For this review, take the finished solid that the model builds, in its own axes (mm). A direction names the side the tool comes from. Coordinates: 2 decimals unless noted, no trailing zeros. Loops run counter-clockwise (first coordinate to the right, second up) from the corner with the lowest first, then second, coordinate; pieces in that order, holes last. Notation, with made-up numbers: (-30.5, -0.5) -> (-18.5, -0.5) arc R16 cw to (-18.5, 16.5) -> close; hole circle Ø7 at (-13, -16.5). An arc over 180 degrees is marked (long way). Answer in a Markdown table with one row per item.
from build123d import *

# Parameters (mm, degrees)
SKETCH1_W           = 99.7966
SKETCH1_H           = 30.1244
BOSS_EXTRUDE1_DEPTH = 2.54
SKETCH2_W           = 33.65475448
SKETCH2_H           = 6.70026545
BOSS_EXTRUDE2_DEPTH = 10.16
SKETCH3_R           = 5.045566178
SKETCH3_W           = 25.4
SKETCH3_H           = 25.4
BOSS_EXTRUDE3_DEPTH = 3.556
FILLET1_R           = 2.54
SKETCH4_R           = 3.429
BOSS_EXTRUDE4_DEPTH = 2.54
FILLET2_R           = 2.54
CHAMFER1_SIZE       = 2.38
SKETCH5_W           = 0.314102564
SKETCH5_H           = 3.5
CUT_EXTRUDE1_DEPTH  = 0.762


with BuildPart() as part:
    # Sketch1 → Boss-Extrude1 (new body)
    with BuildSketch(Plane(origin=(0, 0, 0), x_dir=(1, 0, 0), z_dir=(0, 1, 0))):
        with Locations((49.8983, 15.0622)):
            Rectangle(SKETCH1_W, SKETCH1_H)
    extrude(amount=BOSS_EXTRUDE1_DEPTH)

    # Sketch2 → Boss-Extrude2 (add)
    with BuildSketch(Plane(origin=(0, 2.54, 0), x_dir=(1, 0, 0), z_dir=(0, 1, 0))):
        with Locations((30.013421746, 3.350132725)):
            Rectangle(SKETCH2_W, SKETCH2_H)
    extrude(amount=BOSS_EXTRUDE2_DEPTH)

    # Sketch3 → Boss-Extrude3 (add)
    with BuildSketch(Plane(origin=(0, 2.54, 0), x_dir=(1, 0, 0), z_dir=(0, 1, 0))):
        with Locations(Location((37.834363192, 18.707427202, 0), (0, 0, 90))):
            Circle(SKETCH3_R)
        with Locations((79.4766, 15.0622)):
            Rectangle(SKETCH3_W, SKETCH3_H)
    extrude(amount=BOSS_EXTRUDE3_DEPTH)

    # Fillet1
    fillet1_edges = [part.edges().sort_by_distance(p)[0] for p in [
        (92.1766, 4.318, -27.7622),
        (66.7766, 4.318, -27.7622),
        (66.7766, 4.318, -2.3622),
        (92.1766, 4.318, -2.3622),
    ]]
    fillet(fillet1_edges, radius=FILLET1_R)

    # Sketch4 → Boss-Extrude4 (add)
    with BuildSketch(Plane.ZY):
        with Locations((-15.0622, 0)):
            Circle(SKETCH4_R)
    extrude(amount=BOSS_EXTRUDE4_DEPTH)

    # Fillet2
    fillet2_edges = [part.edges().sort_by_distance(p)[0] for p in [
        (-2.54, 0, -18.4912),
    ]]
    fillet(fillet2_edges, radius=FILLET2_R - 0.0001)  # a hair under: the kernel refuses the full size

    # Chamfer1
    chamfer1_edges = [part.edges().sort_by_distance(p)[0] for p in [
        (30.013421746, 12.7, 0),
    ]]
    chamfer(chamfer1_edges, length=CHAMFER1_SIZE)

    # Sketch5 → Cut-Extrude1 (cut)
    # profile 1 of 7: a face of its own
    with BuildSketch(Plane(origin=(0, 2.54, 0), x_dir=(1, 0, 0), z_dir=(0, 1, 0))):
        Polygon((5.86903585, 16.453640261), (7.484420465, 12.953640261), (7.142974151, 12.953640261), (6.625546267, 14.075435133), (5.038907645, 14.075435133), (4.506756203, 12.953640261), (4.163907645, 12.953640261), (5.824164055, 16.453640261), align=None)
        Polygon((5.843094344, 15.771448755), (5.209280241, 14.434409492), (6.460081523, 14.434409492), align=None, mode=Mode.SUBTRACT)
    # profile 2 of 7: a face of its own
    with BuildSketch(Plane(origin=(0, 2.54, 0), x_dir=(1, 0, 0), z_dir=(0, 1, 0))):
        with Locations((8.269676876, 14.703640261)):
            Rectangle(SKETCH5_W, SKETCH5_H)
    # profile 3 of 7: a face of its own
    with BuildSketch(Plane(origin=(0, 2.54, 0), x_dir=(1, 0, 0), z_dir=(0, 1, 0))):
        Polygon((9.144676876, 12.953640261), (9.606716138, 16.453640261), (9.651587933, 16.453640261), (11.096599953, 13.581845389), (12.538106363, 16.453640261), (12.58367928, 16.453640261), (13.04852303, 12.953640261), (12.733018222, 12.953640261), (12.397882004, 15.472069748), (11.13446053, 12.953640261), (11.063647228, 12.953640261), (9.795317901, 15.477678723), (9.460882805, 12.953640261), align=None)
    # profile 4 of 7: a face of its own
    with BuildSketch(Plane(origin=(0, 2.54, 0), x_dir=(1, 0, 0), z_dir=(0, 1, 0))):
        Polygon((14.865830722, 16.453640261), (15.22831069, 16.453640261), (16.144676876, 15.021949556), (17.061043062, 16.453640261), (17.42352303, 16.453640261), (16.326267421, 14.738696351), (17.468394824, 12.953640261), (17.105914856, 12.953640261), (16.144676876, 14.455443146), (15.183438895, 12.953640261), (14.820958927, 12.953640261), (15.963787453, 14.738696351), align=None)
    # profile 5 of 7: a face of its own
    with BuildSketch(Plane(origin=(0, 2.54, 0), x_dir=(1, 0, 0), z_dir=(0, 1, 0))):
        Polygon((17.670317901, 16.094665902), (17.670317901, 16.453640261), (19.510061491, 16.453640261), (19.510061491, 16.094665902), (18.747240978, 16.094665902), (18.747240978, 12.953640261), (18.433138414, 12.953640261), (18.433138414, 16.094665902), align=None)
    # profile 6 of 7: a face of its own
    with BuildSketch(Plane(origin=(0, 2.54, 0), x_dir=(1, 0, 0), z_dir=(0, 1, 0))):
        with BuildLine():
            Line((20.04852303, 16.453640261), (20.748943703, 16.453640261))
            add(Edge.make_bspline(
                [(20.748943703, 16.453640261), (20.795684831, 16.453484675), (20.885432976, 16.453185933), (21.014006246, 16.45152017), (21.130833343, 16.446745814), (21.235853182, 16.442637231), (21.329063837, 16.435145289), (21.410751128, 16.427984642), (21.480538825, 16.418610981), (21.522784677, 16.409905558), (21.541912453, 16.405963979)],
                knots=[0, 0, 0, 0, 1.410062039, 2.707475311, 3.878576406, 4.937260626, 5.877586885, 6.699081471, 7.410979367, 8, 8, 8, 8], degree=3))
            add(Edge.make_bspline(
                [(21.541912453, 16.405963979), (21.567519077, 16.399637214), (21.618186066, 16.38711865), (21.691136132, 16.360659049), (21.760650456, 16.330039425), (21.826440281, 16.294075704), (21.888176072, 16.252500925), (21.946494383, 16.206032802), (22.001659846, 16.154925596), (22.051441476, 16.097890755), (22.098380528, 16.038054245), (22.137969154, 15.973350488), (22.172095634, 15.905688961), (22.199266151, 15.834381543), (22.221144124, 15.760119771), (22.236570364, 15.682230974), (22.245821551, 15.601069999), (22.246763407, 15.545712091), (22.247240978, 15.517642665)],
                knots=[0, 0, 0, 0, 1.027469482, 2.033020251, 3.019912614, 3.986113645, 4.951240523, 5.91722682, 6.890402269, 7.87763091, 8.8651537, 9.85103654, 10.82876324, 11.815024772, 12.821070561, 13.842952187, 14.906261191, 16, 16, 16, 16], degree=3))
            add(Edge.make_bspline(
                [(22.247240978, 15.517642665), (22.24577198, 15.47100756), (22.242905584, 15.380010392), (22.216180481, 15.247949511), (22.172403961, 15.124760196), (22.112080672, 15.010597558), (22.035261196, 14.907686913), (21.942936405, 14.817296458), (21.835054794, 14.741656545), (21.734625478, 14.68920374), (21.645911278, 14.655610832), (21.572877965, 14.631974473), (21.493210988, 14.613712508), (21.407673653, 14.597352376), (21.315909998, 14.585000682), (21.218139958, 14.575954087), (21.114293807, 14.570300038), (21.042954737, 14.569458033), (21.006255401, 14.569024876)],
                knots=[0, 0, 0, 0, 1.260483769, 2.459530307, 3.627416485, 4.787058657, 5.939039949, 7.08810263, 8.267026773, 9.491475466, 10.141966685, 10.831826277, 11.566392101, 12.351337768, 13.187381173, 14.07005841, 15.007169909, 16, 16, 16, 16], degree=3))
            Line((21.006255401, 14.569024876), (22.292112773, 12.953640261))
            Line((22.292112773, 12.953640261), (21.903691299, 12.953640261))
            Line((21.903691299, 12.953640261), (20.617833927, 14.569024876))
            Line((20.617833927, 14.569024876), (20.362625594, 14.569024876))
            Line((20.362625594, 14.569024876), (20.362625594, 12.953640261))
            Line((20.362625594, 12.953640261), (20.04852303, 12.953640261))
            Line((20.04852303, 12.953640261), (20.04852303, 16.453640261))
        make_face()
        with BuildLine():
            Line((20.362625594, 16.094665902), (20.362625594, 14.927999235))
            Line((20.362625594, 14.927999235), (21.003450914, 14.923091383))
            add(Edge.make_bspline(
                [(21.003450914, 14.923091383), (21.033370953, 14.923078146), (21.09136451, 14.92305249), (21.175265175, 14.927046266), (21.253385287, 14.931589584), (21.325426039, 14.93853893), (21.391419614, 14.947495002), (21.451333027, 14.958697986), (21.505264079, 14.971750048), (21.568162618, 14.991951674), (21.638399149, 15.023957692), (21.714730609, 15.070523191), (21.779732947, 15.12909231), (21.834650809, 15.196065766), (21.87878024, 15.269702015), (21.909892295, 15.349118384), (21.929634737, 15.432309982), (21.931963283, 15.48948809), (21.933138414, 15.518343787)],
                knots=[0, 0, 0, 0, 1.146690395, 2.22261258, 3.21895312, 4.145990853, 4.996080663, 5.770904154, 6.481378293, 7.121626537, 8.300444488, 9.431385265, 10.535395872, 11.636531494, 12.74115979, 13.810798291, 14.895190096, 16, 16, 16, 16], degree=3))
            add(Edge.make_bspline(
                [(21.933138414, 15.518343787), (21.931936293, 15.54649036), (21.929554128, 15.602266599), (21.910105359, 15.683922509), (21.877215978, 15.76098946), (21.83289374, 15.833153945), (21.778894585, 15.89865968), (21.715576772, 15.954706833), (21.644671577, 16.000956298), (21.578400379, 16.030510679), (21.519166166, 16.048630532), (21.467736506, 16.061381696), (21.409625028, 16.071626165), (21.34454957, 16.079834225), (21.272787939, 16.08688917), (21.193977288, 16.091640948), (21.108640508, 16.094454812), (21.049493577, 16.094593901), (21.018875594, 16.094665902)],
                knots=[0, 0, 0, 0, 1.101028733, 2.181837193, 3.264309656, 4.369019818, 5.486613113, 6.575447106, 7.666700264, 8.788928104, 9.402425223, 10.0903467, 10.862060571, 11.710948788, 12.657782767, 13.684531032, 14.801375019, 16, 16, 16, 16], degree=3))
            Line((21.018875594, 16.094665902), (20.362625594, 16.094665902))
        make_face(mode=Mode.SUBTRACT)
    # profile 7 of 7: a face of its own
    with BuildSketch(Plane(origin=(0, 2.54, 0), x_dir=(1, 0, 0), z_dir=(0, 1, 0))):
        Polygon((24.445958927, 16.453640261), (26.061343542, 12.953640261), (25.719897228, 12.953640261), (25.202469344, 14.075435133), (23.615830722, 14.075435133), (23.08367928, 12.953640261), (22.740830722, 12.953640261), (24.401087132, 16.453640261), align=None)
        Polygon((24.420017421, 15.771448755), (23.786203318, 14.434409492), (25.0370046, 14.434409492), align=None, mode=Mode.SUBTRACT)
    extrude(amount=-CUT_EXTRUDE1_DEPTH, mode=Mode.SUBTRACT)

    # Sketch9 → Ø1.5mm Dowel Hole1 (revolve, cut)
    with BuildSketch(Plane(origin=(97.2566, 2.54, -2.54), x_dir=(0, 0, 1), z_dir=(1, 0, 0))):
        Polygon((0, 0), (0, 3.441290929), (1.5, 2.54), (1.5, 0), align=None)
    f_1_5mm_dowel_hole1 = revolve(axis=Axis((97.2566, 8.89, -2.54), (0, -1, 0)), mode=Mode.SUBTRACT)

    # Mirror1: Ø1.5mm Dowel Hole1 across plane
    add(f_1_5mm_dowel_hole1.mirror(Plane.XY.offset(-15.0622)), mode=Mode.SUBTRACT)

    # Mirror2: Ø1.5mm Dowel Hole1 across plane
    add(f_1_5mm_dowel_hole1.mirror(Plane.ZY.offset(-49.8983)), mode=Mode.SUBTRACT)

    # Mirror2 copy 1 sketch → Mirror2 copy 1 (revolve, cut)
    with BuildSketch(Plane(origin=(2.54, 2.54, -27.5844), x_dir=(0, 0, -1), z_dir=(-1, 0, 0))):
        Polygon((0, 0), (0, 3.441290929), (1.5, 2.54), (1.5, 0), align=None)
    revolve(axis=Axis((2.54, 8.89, -27.5844), (0, -1, 0)), mode=Mode.SUBTRACT)


solid = part.part
Item 1: Take a section at A-A, the plane x = 88.5. State the section outline as (y, z) points, and give its area (3 significant figures).
Worked answers:
| item | result |
|---|---|
| outline | (0, -30.12) -> (2.54, -30.12) -> (2.54, -27.76) -> (6.1, -27.76) -> (6.1, -2.36) -> (2.54, -2.36) -> (2.54, 0) -> (0, 0) -> close |
| area | 167 mm² |
Item 2: Take a section at D-D, the plane x = 27. State the section outline as (y, z) points.
Worked answers:
| item | result |
|---|---|
| outline | (0, -30.12) -> (2.54, -30.12) -> (2.54, -6.7) -> (12.7, -6.7) -> (12.7, -2.38) -> (10.32, 0) -> (0, 0) -> close |
Item 3: Insertion check: pin 1 (6 mm diameter, centred on x = 72.5, z = -17, fed in from -Y); pin 2 (2 mm diameter, centred on y = 5.5, z = -25.5, fed in from -X); pin 3 (6 mm diameter, centred on y = 6, z = -8, fed in from +X); pin 4 (0.6 mm diameter, centred on x = 20.5, y = 2, fed in from +Z). Each pin has a flat end and moves straight along its axis. Give the tip position at first contact, or say it passes through.
Worked answers:
| item | result |
|---|---|
| pin 1 | y = 0 |
| pin 2 | x = 66.78 |
| pin 3 | x = 92.18 |
| pin 4 | z = 0 |
Item 4: For L1, parallel to X at y = 1.4, z = -2.54; L2, parallel to Y at x = 21, z = -15.5; L3, parallel to Y at x = 81, z = -23, list the stretches that pass through material, from the lowest coordinate up.
Worked answers:
| item | result |
|---|---|
| L1 | 0 to 1.04, 4.04 to 95.76, 98.76 to 99.8 |
| L2 | 0 to 2.54 |
| L3 | 0 to 6.1 |
Item 5: Take a section at C-C, the plane y = 7.5. State the section outline as (x, z) points.
Worked answers:
| item | result |
|---|---|
| outline | (13.19, -6.7) -> (46.84, -6.7) -> (46.84, 0) -> (13.19, 0) -> close |
Item 6: The part is to be moulded in two halves that separate along X. For faces 1 (the cylindrical face through (91.413, 4.343, -3.087)), 2 (the cylindrical face through (67.54, 4.343, -3.087)), 3 (the flat face through (79, 4, -2.362)), 4 (the cylindrical face through (96, 1.3, -28.4)), say which applies: +X half, -X half, draft (parallel to the pull), parting line (faces both ways), or undercut.
Worked answers:
| item | result |
|---|---|
| face 1 | +X half |
| face 2 | undercut |
| face 3 | draft |
| face 4 | undercut |
Item 7: Take a section at B-B, the plane z = -9.5. State the section outline as (x, y) points.
Worked answers:
| item | result |
|---|---|
| outline | (0, 0) -> (99.8, 0) -> (99.8, 2.54) -> (92.18, 2.54) -> (92.18, 6.1) -> (66.78, 6.1) -> (66.78, 2.54) -> (0, 2.54) -> close |
Item 8: For faces 5 (the flat face through (20.9, 1.778, -14.7)), 6 (the cylindrical face through (91.45, 4.34, -27)), 7 (the flat face through (79, 4, -27.762)), 8 (the flat face through (49, 0, -15)), list the 3-axis set-ups (+Z, -Z, +X, -X, +Y, -Y) from which the entire face can be reached by the end or side of a thin tool; tool diameter is ignored.
Worked answers:
| item | result |
|---|---|
| face 5 | +Y |
| face 6 | -Z, +X, +Y |
| face 7 | -Z, +X, -X, +Y |
| face 8 | +Z, -Z, +X, -Y |
